Design review of the part built by this model. Coordinates are the model's own, in mm. A direction names the side the tool comes from. Coordinates: 2 decimals unless noted, no trailing zeros. Write each loop counter-clockwise with the first axis right and the second up, starting at its lowest first coordinate (ties: lowest second). Pieces come first, ordered by that corner, then holes. Notation, with made-up numbers: (59.5, -36.5) - (96.5, -36.5) arc R25 ccw to (96.5, -20.5) - close; hole circle Ø10 at (-39, 33). An arc over 180 degrees is marked (long way). Use a Markdown table: item, result.
from build123d import *

# Parameters (mm, degrees)
F0_W     = 50
F0_H     = 20
F1_DEPTH = 5
F2_W     = 10
F2_H     = 20
F3_DEPTH = 20
F4_SIZE  = 3
F5_W     = 10
F5_H     = 2
F6_DEPTH = 10
F8_DEPTH = 10
F9_SIZE  = 3


with BuildPart() as f1:
    # F0 (on Top) → F1 (new body)
    with BuildSketch(Plane.XY):
        Rectangle(F0_W, F0_H)
    extrude(amount=F1_DEPTH)

    # F2 (on face) → F3 (join)
    with BuildSketch(Plane.XY.offset(5)):
        with Locations((-20, 0)):
            Rectangle(F2_W, F2_H)
        with Locations((20, 0)):
            Rectangle(F2_W, F2_H)
    extrude(amount=F3_DEPTH)

    # F4
    f4_edges = [f1.edges().sort_by_distance(p)[0] for p in [
        (-15, -10, 15),
        (-15, 10, 15),
        (15, 10, 15),
        (15, -10, 15),
    ]]
    chamfer(f4_edges, length=F4_SIZE)

    # F5 (on face) → F6 (join)
    with BuildSketch(Plane.XY.offset(25)):
        Polygon((-25, -10), (-18, -10), (-15, -7), (-25, -7), align=None)
        with Locations((-20, -6)):
            Rectangle(F5_W, F5_H)
        with Locations((-20, 6)):
            Rectangle(F5_W, F5_H)
        Polygon((-25, 7), (-15, 7), (-18, 10), (-25, 10), align=None)
    extrude(amount=F6_DEPTH)

    # F7 (on face) → F8 (join)
    with BuildSketch(Plane.XY.offset(25)):
        Polygon((25, 10), (18, 10), (15, 7), (15, 5), (25, 5), align=None)
        Polygon((25, -5), (15, -5), (15, -7), (18, -10), (25, -10), align=None)
    extrude(amount=F8_DEPTH)

    # F9
    f9_edges = [f1.edges().sort_by_distance(p)[0] for p in [
        (0, -10, 5),
        (0, 10, 5),
    ]]
    chamfer(f9_edges, length=F9_SIZE)


solid = f1.part
(1) For L1, parallel to X at y = 6.75, z = 16; L2, parallel to Y at x = 19.5, z = 32.5; L3, parallel to X at y = -7.75, z = 6, list the stretches that pass through material, from the lowest coordinate up. Write a range as from..to.
Determined:
| item | result |
|---|---|
| L1 | -25..-15, 15..25 |
| L2 | -10..-5, 5..10 |
| L3 | -25..-15.75, 15.75..25 |
(2) Take a section at A-A on z = 23. Write out the cut boundary in (x, y), and give its area (3 significant figures).
Determined:
| item | result |
|---|---|
| outline | (-25, -10) - (-18, -10) - (-15, -7) - (-15, 7) - (-18, 10) - (-25, 10) - close; (15, -7) - (18, -10) - (25, -10) - (25, 10) - (18, 10) - (15, 7) - close |
| area | 382 mm2 |
(3) Take a section at C-C on y = -0.5. Write out the cut boundary in (x, z).
Determined:
| item | result |
|---|---|
| outline | (-25, 0) - (25, 0) - (25, 25) - (15, 25) - (15, 5) - (-15, 5) - (-15, 25) - (-25, 25) - close |
(4) Draft analysis for pull direction X (two halves, no side actions). For faces 1 (the flat face through (-15, 0, 16)), 2 (the flat face through (16, -8, 18)), 3 (the flat face through (-25, 0, 13)), 4 (the flat face through (0, 10, 1)), state which applies: +X half, -X half, draft (parallel to the pull), parting line (faces both ways), or undercut.
Determined:
| item | result |
|---|---|
| face 1 | undercut |
| face 2 | undercut |
| face 3 | -X half |
| face 4 | draft |
(5) Take a section at D-D on x = 6. Write out the cut boundary in (y, z), and give its area (3 significant figures).
Determined:
| item | result |
|---|---|
| outline | (-10, 0) - (10, 0) - (10, 2) - (7, 5) - (-7, 5) - (-10, 2) - close |
| area | 91.0 mm2 |
(6) Take a section at B-B on x = -21. Write out the cut boundary in (y, z).
Determined:
| item | result |
|---|---|
| outline | (-10, 0) - (10, 0) - (10, 35) - (5, 35) - (5, 25) - (-5, 25) - (-5, 35) - (-10, 35) - close |
(7) For pin 1 (8 mm diameter, centred on x = 17.5, z = 32, fed in from -Y); pin 2 (3 mm diameter, centred on x = -20, y = 1, fed in from +Z); pin 3 (3 mm diameter, centred on x = -6.5, y = -6, fed in from +Z), all flat-tipped, find the tip position at first contact; note any pin that passes through.
Determined:
| item | result |
|---|---|
| pin 1 | y = -10 |
| pin 2 | z = 25 |
| pin 3 | z = 5 |
(8) Machinability: for faces 5 (the flat face through (17, 9, 18)), 6 (the flat face through (20, 5, 30)), 7 (the flat face through (-17, -9, 18)), which of the approach directions +Z, -Z, +X, -X, +Y, -Y give a long, thin tool a straight path to every point of the face, cutting with its end or side? Answer none if there is none.
Determined:
| item | result |
|---|---|
| face 5 | +Z, +Y |
| face 6 | +Z, +X, -X |
| face 7 | +Z, -Y |
